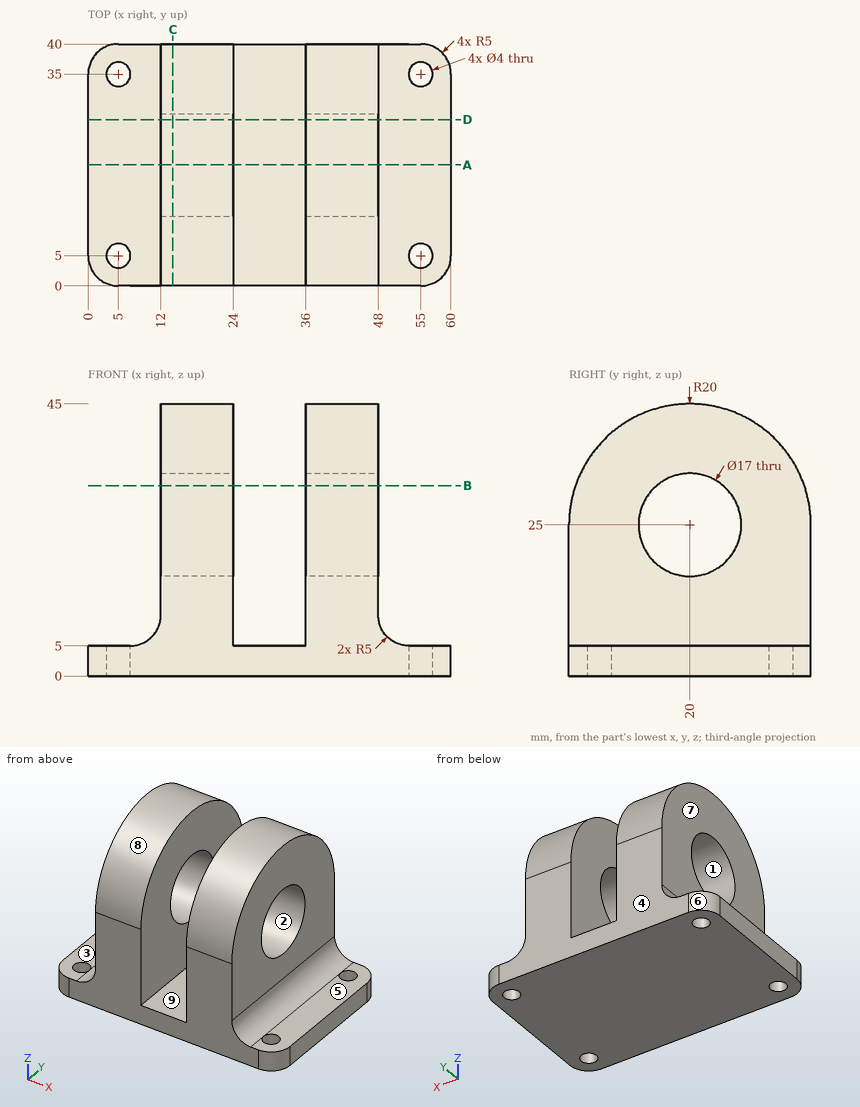
Study the drawing (mm; zero at the part's minimum x, y, z) and answer. A direction names the side the tool comes from. Round coordinates to 2 decimals unless told otherwise and drop trailing zeros. Loops run counter-clockwise (first coordinate to the right, second up) from the corner with the lowest first, then second, coordinate; pieces in that order, holes last. Notation, with made-up numbers: M 40.25,30 L 44.25,30 A21 cw 44.25,35 Z; hole C 79,-25.5 d11. An arc over 180 degrees is marked long. One line per question, with ' | ' between items.
Q1. Consider line 1 along Y through (x, z) = (5, 2); line 2 along X through (y, z) = (26, 16); line 3 along Y through (x, z) = (45, 25). Determine where each line is inside the solid, lowest interval first. Write a range as from..to.
Conclusion:
line 1: y = 0..3, 7..33, 37..40 | line 2: x = 12..24, 36..48 | line 3: y = 0..11.5, 28.5..40
Q2. Find section B-B, the plane z = 31.5. Give the vertices of the cut face in (x, y) (1 decimal).
Conclusion:
outline: M 12,1.1 L 24,1.1 L 24,14.5 L 12,14.5 Z; M 12,25.5 L 24,25.5 L 24,38.9 L 12,38.9 Z; M 36,1.1 L 48,1.1 L 48,14.5 L 36,14.5 Z; M 36,25.5 L 48,25.5 L 48,38.9 L 36,38.9 Z
Q3. Find section A-A, the plane y = 20. Give the vertices of the cut face in (x, z).
Conclusion:
outline: M 0,0 L 60,0 L 60,5 L 53,5 A5 cw 48,10 L 48,16.5 L 36,16.5 L 36,5 L 24,5 L 24,16.5 L 12,16.5 L 12,10 A5 cw 7,5 L 0,5 Z; M 12,33.5 L 24,33.5 L 24,45 L 12,45 Z; M 36,33.5 L 48,33.5 L 48,45 L 36,45 Z
Q4. Find section C-C, the plane x = 14. Give the vertices of the cut face in (y, z).
Conclusion:
outline: M 0,0 L 40,0 L 40,25 A20 ccw 0,25 Z; hole C 20,25 d17
Q5. The mould has two halves that part along Y. Classify the marked faces 1, 2, 3 and 4: +Y half, -Y half, draft (parallel to the pull), parting line (faces both ways), or undercut.
Conclusion:
face 1: undercut | face 2: undercut | face 3: draft | face 4: +Y half
Q6. A tool of negligible diameter and unlimited length cuts with its end or side. For the marked faces 5, 6, 7, 8 and 9, from which of +Z, -Z, +X, -X, +Y, -Y can it reach the whole face along a straight path? Write none if from no direction.
Conclusion:
face 5: +Z, +X, +Y, -Y | face 6: +Z, -Z, -X, +Y | face 7: +Z, -X, +Y, -Y | face 8: +Z, +X, -X | face 9: +Z, +Y, -Y
Q7. Find section D-D, the plane y = 27.5. Give the vertices of the cut face in (x, z).
Conclusion:
outline: M 0,0 L 60,0 L 60,5 L 53,5 A5 cw 48,10 L 48,21 L 36,21 L 36,5 L 24,5 L 24,21 L 12,21 L 12,10 A5 cw 7,5 L 0,5 Z; M 12,29 L 24,29 L 24,43.54 L 12,43.54 Z; M 36,29 L 48,29 L 48,43.54 L 36,43.54 Z
Q8. Each of these flat-tipped pins is pushed along its axis until it touches: pin 1 Ø4 at (y, z) = (8.5, 28) entering from -X; pin 2 Ø5.5 at (x, y) = (4.5, 25.5) entering from +Z; pin 3 Ø19.5 at (y, z) = (20, 25) entering from +X. Where does it stop, or does it pass through?
Conclusion:
pin 1: stops at x = 12 | pin 2: stops at z = 5.01 | pin 3: stops at x = 48
